Input: part model. Units: mm. Frame: model coordinates. A direction names the side the tool comes from. Coordinates: 2 decimals unless noted, no trailing zeros. Write each loop counter-clockwise with the first axis right and the second up, starting at its lowest first coordinate (ties: lowest second). Pieces come first, ordered by that corner, then holes. Notation, with made-up numbers: M -21.5,-38 L -17.5,-38 A5 cw -17.5,-31 Z; hole C 40.25,-38.75 d6. An arc over 180 degrees is marked long. Answer as a JSON object with one key per item and string values. Group by question number.
from build123d import *

# Parameters (mm, degrees)
SKETCH1_R           = 12.5
BOSS_EXTRUDE1_DEPTH = 1
SKETCH2_W           = 3.9
SKETCH2_H           = 3.9
BOSS_EXTRUDE3_DEPTH = 6
SKETCH3_R           = 5
BOSS_EXTRUDE4_DEPTH = 1
BOSS_EXTRUDE5_DEPTH = 6
SKETCH5_R           = 3.204293994
BOSS_EXTRUDE6_DEPTH = 6


with BuildPart() as part:
    # Sketch1 → Boss-Extrude1 (new body, symmetric)
    with BuildSketch(Plane(origin=(0, 0, 0), x_dir=(1, 0, 0), z_dir=(0, 1, 0))):
        Circle(SKETCH1_R)
    extrude(amount=BOSS_EXTRUDE1_DEPTH, both=True)

    # Sketch2 → Boss-Extrude3 (add)
    with BuildSketch(Plane(origin=(0, 1, 0), x_dir=(1, 0, 0), z_dir=(0, 1, 0))):
        with Locations((0, 7.5)):
            Rectangle(SKETCH2_W, SKETCH2_H)
        with Locations((7.5, 0)):
            Rectangle(SKETCH2_W, SKETCH2_H)
        with Locations((0, -7.5)):
            Rectangle(SKETCH2_W, SKETCH2_H)
        with Locations((-7.5, 0)):
            Rectangle(SKETCH2_W, SKETCH2_H)
    extrude(amount=BOSS_EXTRUDE3_DEPTH)

    # Sketch3 → Boss-Extrude4 (add)
    with BuildSketch(Plane.XZ.offset(1)):
        Circle(SKETCH3_R)
    extrude(amount=BOSS_EXTRUDE4_DEPTH)

    # Sketch4 → Boss-Extrude5 (add)
    with BuildSketch(Plane.XZ.offset(2)):
        Polygon((0, -3.7), (3.204293994, -1.85), (3.204293994, 1.85), (0, 3.7), (-3.204293994, 1.85), (-3.204293994, -1.85), align=None)
    extrude(amount=BOSS_EXTRUDE5_DEPTH)

    # Sketch5 → Boss-Extrude6 (add)
    with BuildSketch(Plane(origin=(0, -8, 0), x_dir=(-1, 0, 0), z_dir=(0, -1, 0))):
        Circle(SKETCH5_R)
    extrude(amount=BOSS_EXTRUDE6_DEPTH)


solid = part.part
Q1. Section B-B, the plane z = 6.5. Return the cut outline in (x, y), and give its area (3 significant figures).
Q2. Draft query along X for faces 1 (the cylindrical face through (11.923, 0.014, -3.755)), 2 (the flat face through (-1.95, 4, 8)), 3 (the flat face through (-5.55, 4, 0)), 4 (the flat face through (0, -8, 3.4)). Return one class per face: released by +X, released by -X, zero draft, split by the parting line, or undercut.
Q3. Section A-A, the plane y = 2.75. Return the cut outline in (x, z).
Q4. Line query: line 1 (Y direction, x = -2.75, z = 5); line 2 (Y direction, x = -2.5, z = 1.25); line 3 (Z direction, x = 0, y = 3.5). Output: solid intervals per line, ascending. Write a range as from..to.
Q5. Pin query (flat end, axial travel): pin 1 Ø3 at (y, z) = (4.5, -8) entering from +X; pin 2 Ø12.5 at (x, z) = (-1.5, -5) entering from +Y; pin 3 Ø3 at (y, z) = (-9, 0.5) entering from +X; pin 4 Ø2 at (y, z) = (4, 1) entering from +X. Return the tip coordinate at first contact, or that it passes through.
Q6. Section D-D, the plane y = -4.25. Return the cut outline in (x, z).
Q7. Access query for faces 5 (the flat face through (2.9, -8, 1.7)), 6 (the cylindrical face through (2.543, -10.958, 1.95)), 7 (the flat face through (9.45, 4, 0)), 8 (the flat face through (-3.204, -5, 0)). Directions: +Z, -Z, +X, -X, +Y, -Y. A direction counts if a zero-diameter tool reaches every point of the face in a straight line with its end or side. Return the directions, or none.
Q8. Section C-C, the plane x = -0.5. Return the cut outline in (y, z).
Filled in:
{
 "1": {"outline": "M -10.68,-1 L 10.68,-1 L 10.68,1 L 1.95,1 L 1.95,7 L -1.95,7 L -1.95,1 L -10.68,1 Z", "area": "66.1 mm^2"},
 "2": {"face 1": "split by the parting line", "face 2": "released by -X", "face 3": "undercut", "face 4": "zero draft"},
 "3": {"outline": "M -9.45,-1.95 L -5.55,-1.95 L -5.55,1.95 L -9.45,1.95 Z; M -1.95,-9.45 L 1.95,-9.45 L 1.95,-5.55 L -1.95,-5.55 Z; M -1.95,5.55 L 1.95,5.55 L 1.95,9.45 L -1.95,9.45 Z; M 5.55,-1.95 L 9.45,-1.95 L 9.45,1.95 L 5.55,1.95 Z"},
 "4": {"line 1": "-1..1", "line 2": "-14..1", "line 3": "-9.45..-5.55, 5.55..9.45"},
 "5": {"pin 1": "x = 1.95", "pin 2": "y = 7", "pin 3": "x = 3.2", "pin 4": "x = 9.45"},
 "6": {"outline": "M -3.2,-1.85 L 0,-3.7 L 3.2,-1.85 L 3.2,1.85 L 0,3.7 L -3.2,1.85 Z"},
 "7": {"face 5": "+Z, +X, -Y", "face 6": "-Y", "face 7": "+Z, -Z, +X, +Y", "face 8": "+Z, -Z, -X, -Y"},
 "8": {"outline": "M -14,-3.17 L -8,-3.17 L -8,-3.41 L -2,-3.41 L -2,-4.97 L -1,-4.97 L -1,-12.49 L 1,-12.49 L 1,-9.45 L 7,-9.45 L 7,-5.55 L 1,-5.55 L 1,5.55 L 7,5.55 L 7,9.45 L 1,9.45 L 1,12.49 L -1,12.49 L -1,4.97 L -2,4.97 L -2,3.41 L -8,3.41 L -8,3.17 L -14,3.17 Z"}
}
